from build123d import *

# Parameters (mm, degrees)
F1_DEPTH       = 270
F2_T           = -7
F5_D           = 5
F5_DEPTH       = 20
F5_CBORE_D     = 10
F5_CBORE_DEPTH = 5
F6_R           = 5


with BuildPart() as f1:
    # F0 (on Front) → F1 (new body)
    with BuildSketch(Plane.XZ):
        Polygon((37.060434, -74.633442), (76.363391, -33.350546), (79.93507, 23.537441), (46.10424, 69.411998), (-9.299275, 82.80791), (-60.351557, 57.45708), (-83.164674, 5.221444), (-67.064116, -49.457364), (-19.583513, -80.994521), align=None)
    extrude(amount=F1_DEPTH)

    # F2
    f2_openings = [f1.faces().sort_by_distance(p)[0] for p in [
        (0, -270, 0),
    ]]
    offset(amount=F2_T, openings=f2_openings)

    # F5
    with Locations(Plane(origin=(8.73846, 0, -77.813982), x_dir=(0.993753, 0, 0.111598), z_dir=(0.111598, 0, -0.993753))):
        with Locations((0, 190.445736)):
            CounterBoreHole(F5_D / 2, F5_CBORE_D / 2, F5_CBORE_DEPTH, depth=F5_DEPTH)

    # F6
    f6_edges = [f1.edges().sort_by_distance(p)[0] for p in [
        (-75.114395, -270, -22.11796),
        (8.73846, -270, -77.813982),
        (56.711913, -270, -53.991994),
        (-43.323814, -270, -65.225943),
        (78.14923, -270, -4.906553),
        (63.019655, -270, 46.47472),
        (18.402482, -270, 76.109954),
        (-34.825416, -270, 70.132495),
        (-71.758115, -270, 31.339262),
    ]]
    fillet(f6_edges, radius=F6_R)


solid = f1.part
Could you check a few things on this model? Use its own coordinates, in mm. A direction names the side the tool comes from. Coordinates: 2 decimals unless noted, no trailing zeros. Write each loop counter-clockwise with the first axis right and the second up, starting at its lowest first coordinate (ties: lowest second). Pieces come first, ordered by that corner, then holes. Notation, with made-up numbers: (11.25, 59) - (19.25, 59) arc R30 cw to (19.25, 98) - close; hole circle Ø5 at (-15.75, 41). An arc over 180 degrees is marked (long way). Put each result on its own line as item: value. Start each with the question number.
Q1. Thinking about a two-plate mould opening in X: for faces 1 (the flat face through (17.11, -136.66, 69.22)), 2 (the cylindrical face through (55.95, -268.5, -52.72)), 3 (the flat face through (-3, 0, 2)), which applies, pulls with the +X half, pulls with the -X half, needs draft (parallel to the pull), parting line crosses it, or undercut?
Q2. I want a section at A-A on y = -51.5. Write out the boundary of the cut face in (x, z), plus the area to 3 significant figures.
Q3. Please list where these lines run through material, in increasing order: L1, parallel to X at y = -58, z = -11; L2, parallel to X at y = -193, z = 8.5; L3, parallel to Z at x = 61, y = -137.
Q4. I'm going to push flat-ended pins straight in: P1, Ø3, axis at x = -52.5, y = -43, coming from the -Z side; P2, Ø3, axis at x = 9, y = -31.5, coming from the +Z side; P3, Ø6, axis at x = -32, y = -72, coming from the -Z side. Where does each tip first touch, or does it pass through?
Q5. Which directions (+Z, -Z, +X, -X, +Y, -Y) give clear straight access to the entire face, cutting with the end or side of a thin tool? Please do faces 4 (the flat face through (-68.5, -136.7, -19.8)), 5 (the cylindrical face through (10.76, -186.01, -75.11)).
Checks:
1. face 1: undercut
1. face 2: pulls with the +X half
1. face 3: needs draft
2. outline: (-83.16, 5.22) - (-67.06, -49.46) - (-19.58, -80.99) - (37.06, -74.63) - (76.36, -33.35) - (79.94, 23.54) - (46.1, 69.41) - (-9.3, 82.81) - (-60.35, 57.46) - close; hole (-75.73, 4.75) - (-61.07, -45.04) - (-17.83, -73.75) - (33.75, -67.96) - (69.54, -30.37) - (72.79, 21.43) - (41.98, 63.21) - (-8.47, 75.41) - (-54.96, 52.32) - close
2. area: 3,430 mm²
3. L1: -78.39 to -71.09, 70.75 to 77.77
3. L2: -81.73 to -74.09, 71.98 to 78.99
3. L3: -49.49 to -39.34, 37.42 to 49.21
4. P1: z = -60.13
4. P2: z = 78.75
4. P3: z = -74.74
5. face 4: -Y
5. face 5: none
